Source: CAD feature listing. Evaluate the final solid. Frame: model axes, mm. Face numbers are marked on the shaded views. Give positions to 0.01 mm unless a question says otherwise; leave off trailing zeros. Write each loop counter-clockwise with the first axis right and the second up, starting at its lowest first coordinate (ties: lowest second). Pieces come first, ordered by that corner, then holes. Notation, with made-up numbers: (78.5, 4) -> (104.5, 4) arc R9 cw to (104.5, 12) -> close; hole circle Ø6 at (-23, 5.25). An arc over 180 degrees is marked (long way). Answer as a JSON object with one key per item and string values. Group by question number.
Item 1: Section query B-B on z = 26. Return the cut outline in (x, y), plus the area to 3 significant figures.
Item 2: Ray query, probe 1 along X at (y, z) = (0.25, 29); probe 2 along Z at (x, y) = (24.5, -1.25); probe 3 along Y at (x, z) = (24, -5.5). Return the intervals inside material, ascending. Write a range as from..to.
Item 3: Pull-direction query (Z, two-part tool) for the marked faces 1 and 2; classes: pulls with the +Z half, pulls with the -Z half, needs draft (parallel to the pull), parting line crosses it, or undercut.
Item 4: Section query D-D on x = -19.5. Return the cut outline in (y, z), plus the area to 3 significant figures.
Item 5: Section query A-A on y = -1.75. Return the cut outline in (x, z), plus the area to 3 significant figures.
Item 6: Section query C-C on x = 1.5. Return the cut outline in (y, z) (3 decimals).
from build123d import *

# Parameters (mm, degrees)
EXTRUDE_1_DEPTH     = 4
EXTRUDE_2_DEPTH     = 4
SKETCH_3_R          = 1.25
CUT_EXTRUDE_1_DEPTH = 15
CUT_EXTRUDE_2_DEPTH = 0.2
EXTRUDE_5_DEPTH     = 0.2
EXTRUDE_6_DEPTH     = 0.2
SKETCH_13_R         = 2.280555424
SKETCH_13_R_2       = 2.93479419
SKETCH_13_R_3       = 2.630805897
SKETCH_13_R_4       = 2.84821008
EXTRUDE_7_DEPTH     = 0.2


with BuildPart() as part:
    # 草图1 → 凸台-拉伸1 (new body)
    with BuildSketch(Plane(origin=(0, 0, 0), x_dir=(1, 0, 0), z_dir=(0, 1, 0))):
        with BuildLine():
            Line((-27.00005461, -31.987363475), (27.00005461, -31.987363475))
            ThreePointArc((27.00005461, -31.987363475), (29.112398272, -31.112402082), (29.987359665, -29.00005842))
            Line((29.987359665, -29.00005842), (29.987359665, 29.00005842))
            ThreePointArc((29.987359665, 29.00005842), (29.112398272, 31.112402082), (27.00005461, 31.987363475))
            Line((27.00005461, 31.987363475), (-27.00005461, 31.987363475))
            ThreePointArc((-27.00005461, 31.987363475), (-29.112398272, 31.112402082), (-29.987359665, 29.00005842))
            Line((-29.987359665, 29.00005842), (-29.987359665, -29.00005842))
            ThreePointArc((-29.987359665, -29.00005842), (-29.112398272, -31.112402082), (-27.00005461, -31.987363475))
        make_face()
    extrude(amount=EXTRUDE_1_DEPTH)

    # 草图2 → 凸台-拉伸2 (add)
    with BuildSketch(Plane.XZ):
        with BuildLine():
            Line((-21.987359665, 23.987363475), (-21.987359665, 31.987363475))
            Line((-21.987359665, 31.987363475), (-27.00005461, 31.987363475))
            ThreePointArc((-27.00005461, 31.987363475), (-29.112398272, 31.112402082), (-29.987359665, 29.00005842))
            Line((-29.987359665, 29.00005842), (-29.987359665, 23.987363475))
            Line((-29.987359665, 23.987363475), (-21.987359665, 23.987363475))
        make_face()
        with BuildLine():
            Line((21.987359665, -23.987363475), (21.987359665, -31.987363475))
            Line((21.987359665, -31.987363475), (27.00005461, -31.987363475))
            ThreePointArc((27.00005461, -31.987363475), (29.112398272, -31.112402082), (29.987359665, -29.00005842))
            Line((29.987359665, -29.00005842), (29.987359665, -23.987363475))
            Line((29.987359665, -23.987363475), (21.987359665, -23.987363475))
        make_face()
        with BuildLine():
            Line((21.987359665, 23.987363475), (29.987359665, 23.987363475))
            Line((29.987359665, 23.987363475), (29.987359665, 29.00005842))
            ThreePointArc((29.987359665, 29.00005842), (29.112398272, 31.112402082), (27.00005461, 31.987363475))
            Line((27.00005461, 31.987363475), (21.987359665, 31.987363475))
            Line((21.987359665, 31.987363475), (21.987359665, 23.987363475))
        make_face()
        with BuildLine():
            Line((-29.987359665, -23.987363475), (-29.987359665, -29.00005842))
            ThreePointArc((-29.987359665, -29.00005842), (-29.112398272, -31.112402082), (-27.00005461, -31.987363475))
            Line((-27.00005461, -31.987363475), (-21.987359665, -31.987363475))
            Line((-21.987359665, -31.987363475), (-21.987359665, -23.987363475))
            Line((-21.987359665, -23.987363475), (-29.987359665, -23.987363475))
        make_face()
    extrude(amount=EXTRUDE_2_DEPTH)

    # 草图3 → 切除-拉伸1 (cut)
    with BuildSketch(Plane.XZ.offset(4)):
        with Locations(Location((-27.00005461, 29.00005842, 0), (0, 0, 270))):
            Circle(SKETCH_3_R)
        with Locations(Location((27.00005461, 29.00005842, 0), (0, 0, 270))):
            Circle(SKETCH_3_R)
        with Locations(Location((27.00005461, -29.00005842, 0), (0, 0, 270))):
            Circle(SKETCH_3_R)
        with Locations(Location((-27.00005461, -29.00005842, 0), (0, 0, 270))):
            Circle(SKETCH_3_R)
    extrude(amount=-CUT_EXTRUDE_1_DEPTH, mode=Mode.SUBTRACT)

    # 草图4 → 切除-拉伸2 (cut)
    with BuildSketch(Plane(origin=(0, 4, 0), x_dir=(1, 0, 0), z_dir=(0, 1, 0))):
        with BuildLine():
            Line((-22, -25), (22, -25))
            ThreePointArc((22, -25), (24.121320344, -24.121320344), (25, -22))
            Line((25, -22), (25, 22))
            ThreePointArc((25, 22), (24.121320344, 24.121320344), (22, 25))
            Line((22, 25), (-22, 25))
            ThreePointArc((-22, 25), (-24.121320344, 24.121320344), (-25, 22))
            Line((-25, 22), (-25, -22))
            ThreePointArc((-25, -22), (-24.121320344, -24.121320344), (-22, -25))
        make_face()
    extrude(amount=-CUT_EXTRUDE_2_DEPTH, mode=Mode.SUBTRACT)

    # 草图9 → 凸台-拉伸5 (add)
    with BuildSketch(Plane(origin=(0, 3.8, 0), x_dir=(1, 0, 0), z_dir=(0, 1, 0))):
        with BuildLine():
            ThreePointArc((-21.208751083, 8.458751083), (-20.987642877, 8.127839267), (-20.91, 7.737502166))
            Line((-20.91, 7.737502166), (-20.91, -7.737502166))
            ThreePointArc((-20.91, -7.737502166), (-20.987642877, -8.127839267), (-21.208751083, -8.458751083))
            Line((-21.208751083, -8.458751083), (-22.850416306, -10.100416306))
            ThreePointArc((-22.850416306, -10.100416306), (-22.924119041, -10.210720244), (-22.95, -10.340832611))
            Line((-22.95, -10.340832611), (-22.95, -19.409167389))
            ThreePointArc((-22.95, -19.409167389), (-22.924119041, -19.539279756), (-22.850416306, -19.649583694))
            Line((-22.850416306, -19.649583694), (-21.349583694, -21.150416306))
            ThreePointArc((-21.349583694, -21.150416306), (-21.239279756, -21.224119041), (-21.109167389, -21.25))
            Line((-21.109167389, -21.25), (21.109167389, -21.25))
            ThreePointArc((21.109167389, -21.25), (21.239279756, -21.224119041), (21.349583694, -21.150416306))
            Line((21.349583694, -21.150416306), (22.850416306, -19.649583694))
            ThreePointArc((22.850416306, -19.649583694), (22.924119041, -19.539279756), (22.95, -19.409167389))
            Line((22.95, -19.409167389), (22.95, -10.340832611))
            ThreePointArc((22.95, -10.340832611), (22.924119041, -10.210720244), (22.850416306, -10.100416306))
            Line((22.850416306, -10.100416306), (21.208751083, -8.458751083))
            ThreePointArc((21.208751083, -8.458751083), (20.987642877, -8.127839267), (20.91, -7.737502166))
            Line((20.91, -7.737502166), (20.91, 7.737502166))
            ThreePointArc((20.91, 7.737502166), (20.987642877, 8.127839267), (21.208751083, 8.458751083))
            Line((21.208751083, 8.458751083), (22.850416306, 10.100416306))
            ThreePointArc((22.850416306, 10.100416306), (22.924119041, 10.210720244), (22.95, 10.340832611))
            Line((22.95, 10.340832611), (22.95, 19.409167389))
            ThreePointArc((22.95, 19.409167389), (22.924119041, 19.539279756), (22.850416306, 19.649583694))
            Line((22.850416306, 19.649583694), (21.349583694, 21.150416306))
            ThreePointArc((21.349583694, 21.150416306), (21.239279756, 21.224119041), (21.109167389, 21.25))
            Line((21.109167389, 21.25), (-21.109167389, 21.25))
            ThreePointArc((-21.109167389, 21.25), (-21.239279756, 21.224119041), (-21.349583694, 21.150416306))
            Line((-21.349583694, 21.150416306), (-22.850416306, 19.649583694))
            ThreePointArc((-22.850416306, 19.649583694), (-22.924119041, 19.539279756), (-22.95, 19.409167389))
            Line((-22.95, 19.409167389), (-22.95, 10.340832611))
            ThreePointArc((-22.95, 10.340832611), (-22.924119041, 10.210720244), (-22.850416306, 10.100416306))
            Line((-22.850416306, 10.100416306), (-21.208751083, 8.458751083))
        make_face()
        with BuildLine():
            ThreePointArc((-14.688, -17.765), (-16.15, -19.227), (-17.612, -17.765))
            ThreePointArc((-17.612, -17.765), (-16.15, -16.303), (-14.688, -17.765))
        make_face(mode=Mode.SUBTRACT)
        with BuildLine():
            ThreePointArc((14.688, -17.765), (16.15, -16.303), (17.612, -17.765))
            ThreePointArc((17.612, -17.765), (16.15, -19.227), (14.688, -17.765))
        make_face(mode=Mode.SUBTRACT)
        with BuildLine():
            Line((11.9, -12.495), (-11.9, -12.495))
            ThreePointArc((-11.9, -12.495), (-13.522810063, -11.822810063), (-14.195, -10.2))
            Line((-14.195, -10.2), (-14.195, 10.2))
            ThreePointArc((-14.195, 10.2), (-13.522810063, 11.822810063), (-11.9, 12.495))
            Line((-11.9, 12.495), (11.9, 12.495))
            ThreePointArc((11.9, 12.495), (13.522810063, 11.822810063), (14.195, 10.2))
            Line((14.195, 10.2), (14.195, -10.2))
            ThreePointArc((14.195, -10.2), (13.522810063, -11.822810063), (11.9, -12.495))
        make_face(mode=Mode.SUBTRACT)
        with BuildLine():
            ThreePointArc((-14.688, 17.765), (-16.15, 16.303), (-17.612, 17.765))
            ThreePointArc((-17.612, 17.765), (-16.15, 19.227), (-14.688, 17.765))
        make_face(mode=Mode.SUBTRACT)
        with BuildLine():
            ThreePointArc((17.612, 17.765), (16.15, 16.303), (14.688, 17.765))
            ThreePointArc((14.688, 17.765), (16.15, 19.227), (17.612, 17.765))
        make_face(mode=Mode.SUBTRACT)
    extrude(amount=EXTRUDE_5_DEPTH)

    # 草图12 → 凸台-拉伸6 (add)
    with BuildSketch(Plane(origin=(0, 3.8, 0), x_dir=(1, 0, 0), z_dir=(0, 1, 0))):
        Polygon((5.362596469, -4.798672993), (5.362596469, -2.219483683), (3.321803619, -2.219483683), (3.321803619, 8.634725488), (-0.595580356, 8.634725488), (-7.046362352, -2.587805787), (-7.046362352, -4.798672993), (0.108141316, -4.798672993), (0.108141316, -9.18520475), (3.321803619, -9.18520475), (3.321803619, -4.798672993), align=None)
        with BuildLine():
            add(Edge.make_bspline(
                [(-1.346216807, 2.419233234), (-1.215389858, 2.676405088), (-0.953971645, 3.190285503), (-0.591881771, 3.983382076), (-0.22871235, 4.799127855), (0.024319607, 5.348664428), (0.153889522, 5.630065273)],
                knots=[0, 0, 0, 0, 0.976764423, 1.951769216, 2.951163759, 4, 4, 4, 4], degree=3))
            Line((0.153889522, 5.630065273), (0.248885651, 5.632179686))
            add(Edge.make_bspline(
                [(0.248885651, 5.632179686), (0.211585261, 5.077369517), (0.137462974, 3.974866313), (0.116695103, 2.87007222), (0.106378201, 2.321241135)],
                knots=[0, 0, 0, 0, 1.006455431, 2, 2, 2, 2], degree=3))
            Line((0.106378201, 2.321241135), (0.108141316, -2.219483683))
            Line((0.108141316, -2.219483683), (-3.949986994, -2.219483683))
            Line((-3.949986994, -2.219483683), (-3.949986994, -2.171163716))
            Line((-3.949986994, -2.171163716), (-1.346216807, 2.419233234))
        make_face(mode=Mode.SUBTRACT)
    extrude(amount=EXTRUDE_6_DEPTH)

    # 草图13 → 凸台-拉伸7 (add)
    with BuildSketch(Plane(origin=(0, 3.8, 0), x_dir=(1, 0, 0), z_dir=(0, 1, 0))):
        with Locations((-16.15, 17.765)):
            Circle(SKETCH_13_R)
        with Locations((16.15, 17.765)):
            Circle(SKETCH_13_R_2)
        with Locations((16.15, -17.765)):
            Circle(SKETCH_13_R_3)
        with Locations((-16.15, -17.765)):
            Circle(SKETCH_13_R_4)
    extrude(amount=EXTRUDE_7_DEPTH)


solid = part.part
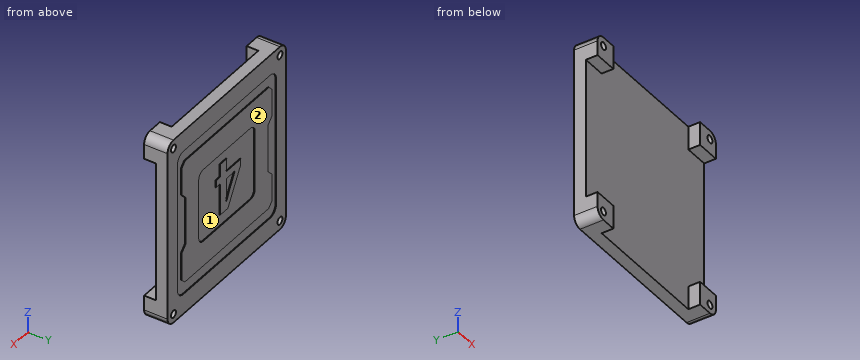
Worked answers:
{
 "1": {"outline": "(-29.99, -4) -> (-21.99, -4) -> (-21.99, 0) -> (21.99, 0) -> (21.99, -4) -> (29.99, -4) -> (29.99, 4) -> (-29.99, 4) -> close", "area": "304 mm^2"},
 "2": {"probe 1": "-29.99..-28.25, -25.75..25.75, 28.25..29.99", "probe 2": "-31.99..-23.99, 23.99..31.99", "probe 3": "0..3.8"},
 "3": {"face 1": "undercut", "face 2": "needs draft"},
 "4": {"outline": "(0, -31.99) -> (4, -31.99) -> (4, -25) -> (3.8, -25) -> (3.8, -21.25) -> (4, -21.25) -> (4, 21.25) -> (3.8, 21.25) -> (3.8, 25) -> (4, 25) -> (4, 31.99) -> (0, 31.99) -> close", "area": "254 mm^2"},
 "5": {"outline": "(-29.99, -29) arc R2.99 ccw to (-27, -31.99) -> (-21.99, -31.99) -> (-21.99, -23.99) -> (-29.99, -23.99) -> close; (-29.99, 23.99) -> (-21.99, 23.99) -> (-21.99, 31.99) -> (-27, 31.99) arc R2.99 ccw to (-29.99, 29) -> close; (21.99, -31.99) -> (27, -31.99) arc R2.99 ccw to (29.99, -29) -> (29.99, -23.99) -> (21.99, -23.99) -> close; (21.99, 23.99) -> (29.99, 23.99) -> (29.99, 29) arc R2.99 ccw to (27, 31.99) -> (21.99, 31.99) -> close; hole circle Ø2.5 at (-27, -29); hole circle Ø2.5 at (-27, 29); hole circle Ø2.5 at (27, -29); hole circle Ø2.5 at (27, 29)", "area": "229 mm^2"},
 "6": {"outline": "(0, -31.987) -> (4, -31.987) -> (4, -25) -> (3.8, -25) -> (3.8, -21.25) -> (4, -21.25) -> (4, -12.495) -> (3.8, -12.495) -> (3.8, -8.635) -> (4, -8.635) -> (4, 9.185) -> (3.8, 9.185) -> (3.8, 12.495) -> (4, 12.495) -> (4, 21.25) -> (3.8, 21.25) -> (3.8, 25) -> (4, 25) -> (4, 31.987) -> (0, 31.987) -> close"}
}
